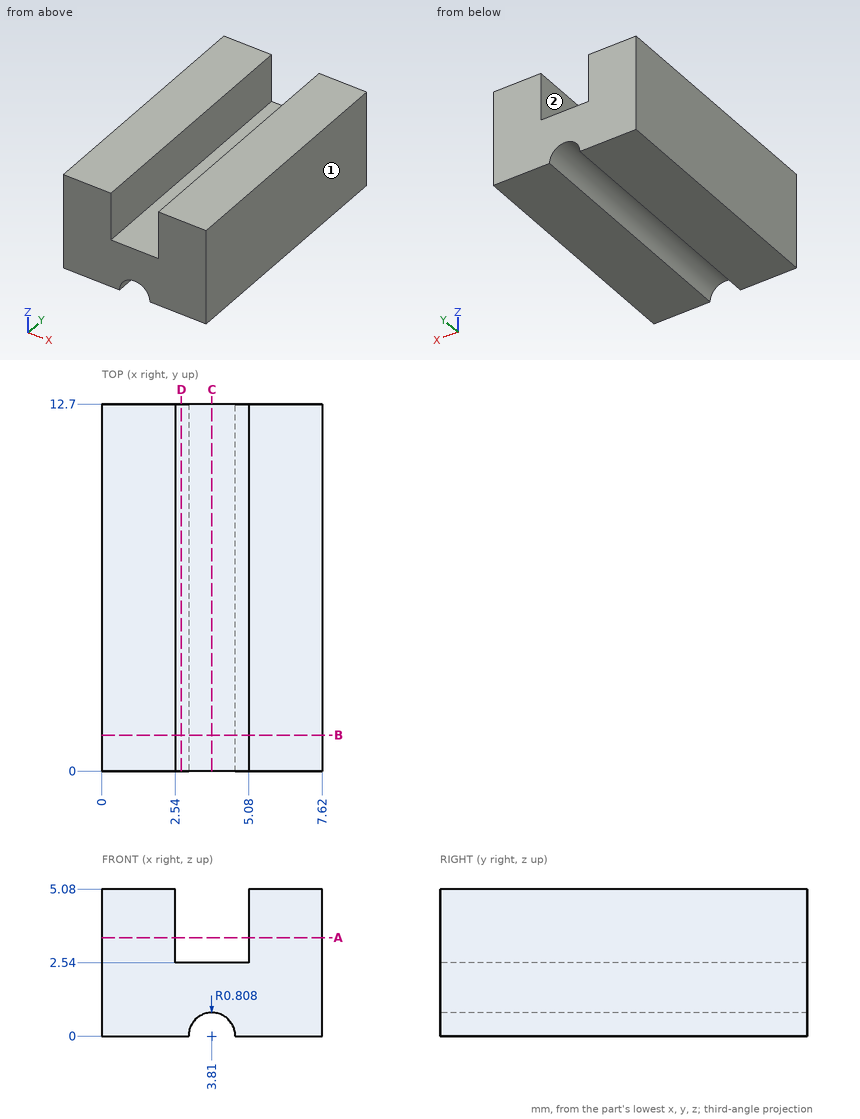
Geometry check sheet. Reference: drawing and pictorial views, mm from the part's lowest x, y, z. A direction names the side the tool comes from. Give positions to 0.01 mm unless a question says otherwise; leave off trailing zeros. Loops run counter-clockwise (first coordinate to the right, second up) from the corner with the lowest first, then second, coordinate; pieces in that order, holes last.
1. Section check B-B, the plane y = 1.25. Enter the section's corners in (x, z).
2. Go/stop test with a flat-tipped pin: pin 1 Ø0.8 at (x, y) = (3.5, 4) entering from +Z. Record where the tip stops, or that it passes through.
3. Thickness scan on line 1 (X direction, y = 7, z = 3.1); line 2 (X direction, y = 7.25, z = 0.2); line 3 (Z direction, x = 4.25, y = 4.5). Record the ranges inside material, lowest first.
4. Section check D-D, the plane x = 2.75. Enter the section's corners in (y, z).
5. Section check A-A, the plane z = 3.4. Enter the section's corners in (x, y).
6. Set-up check for the marked faces 1 and 2: record each of +Z, -Z, +X, -X, +Y, -Y from which the full face is reachable in a straight line by a thin tool's end or side.
7. Section check C-C, the plane x = 3.81. Enter the section's corners in (y, z), then the cut area to 3 significant figures.
Geometry says:
1. outline: (0, 0) - (3, 0) arc R0.81 cw to (4.62, 0) - (7.62, 0) - (7.62, 5.08) - (5.08, 5.08) - (5.08, 2.54) - (2.54, 2.54) - (2.54, 5.08) - (0, 5.08) - close
2. pin 1: stops at z = 2.54
3. line 1: x = 0 to 2.54, 5.08 to 7.62
3. line 2: x = 0 to 3.03, 4.59 to 7.62
3. line 3: z = 0.68 to 2.54
4. outline: (0, 0) - (12.7, 0) - (12.7, 2.54) - (0, 2.54) - close
5. outline: (0, 0) - (2.54, 0) - (2.54, 12.7) - (0, 12.7) - close; (5.08, 0) - (7.62, 0) - (7.62, 12.7) - (5.08, 12.7) - close
6. face 1: +Z, -Z, +X, +Y, -Y
6. face 2: +Z, +Y, -Y
7. outline: (0, 0.81) - (12.7, 0.81) - (12.7, 2.54) - (0, 2.54) - close
7. area: 22.0 mm2
